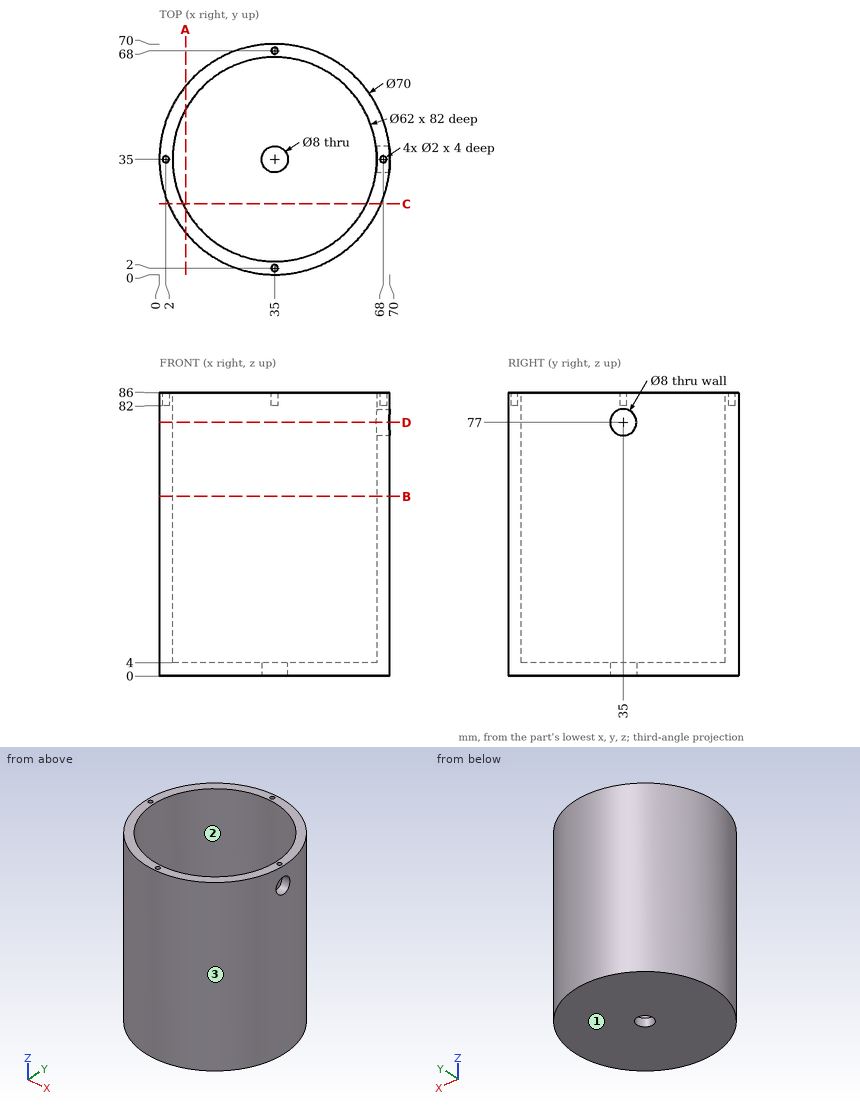
Input: dimensioned drawing with shaded views. Units: mm. Origin: part minimum x, y, z. Round coordinates to 2 decimals unless told otherwise and drop trailing zeros. Loops run counter-clockwise (first coordinate to the right, second up) from the corner with the lowest first, then second, coordinate; pieces in that order, holes last. Notation, with made-up numbers: M 85,-25 L 109,-25 A27 cw 109,-1 Z; hole C 32.25,22 d11. An arc over 180 degrees is marked long. Answer in a Markdown table with one row per item. Add a question column.
1. Contact query for flat-ended pins moving along their axis: pin 1 (6 mm diameter, centred on y = 23, z = 61, fed in from +X); pin 2 (0.6 mm diameter, centred on x = 2, y = 34.5, fed in from +Z); pin 3 (10 mm diameter, centred on x = 26, y = 52.5, fed in from +Z). Output: stop coordinate, or through.
2. Section C-C (y = 21.5). Output: boundary loops of the cut face in (x, z), and give its area (3 significant figures).
3. Ray query, probe 1 along X at (y, z) = (35.5, 27); probe 2 along X at (y, z) = (56, 6); probe 3 along Z at (x, y) = (16.5, 48.5). Return the intervals inside material, ascending.
4. Section D-D (z = 77). Output: boundary loops of the cut face in (x, y), and give its area (3 significant figures).
5. Mould query, pull axis Y, two halves, no side actions, for the marked faces 1, 2 and 3. Classes: released by +Y, released by -Y, zero draft, split by the parting line, or undercut.
6. Section A-A (x = 8). Output: boundary loops of the cut face in (y, z), and give its area (3 significant figures).
7. Section B-B (z = 54.5). Output: boundary loops of the cut face in (x, y).
Values follow:
| question | item | result |
|---|---|---|
| 1 | pin 1 | x = 68.82 |
| 1 | pin 2 | z = 82 |
| 1 | pin 3 | z = 4 |
| 2 | outline | M 2.71,0 L 67.29,0 L 67.29,86 L 62.91,86 L 62.91,4 L 7.09,4 L 7.09,86 L 2.71,86 Z |
| 2 | area | 978 mm^2 |
| 3 | probe 1 | 0 to 4, 66 to 70 |
| 3 | probe 2 | 7 to 12.2, 57.8 to 63 |
| 3 | probe 3 | 0 to 4 |
| 4 | outline | M 65.74,31 A31 cw long 65.74,39 L 69.77,39 A35 ccw long 69.77,31 Z |
| 4 | area | 797 mm^2 |
| 5 | face 1 | zero draft |
| 5 | face 2 | undercut |
| 5 | face 3 | split by the parting line |
| 6 | outline | M 12.73,0 L 57.27,0 L 57.27,86 L 50.23,86 L 50.23,4 L 19.77,4 L 19.77,86 L 12.73,86 Z |
| 6 | area | 1,330 mm^2 |
| 7 | outline | C 35,35 d70; hole C 35,35 d62 |
